The figure shows three views and two pictorial views of one solid part (mm, origin at its lowest corner). Answer the questions. Give positions to 0.01 mm unless a question says otherwise; leave off trailing zeros. Order: outer loops, then holes, each group sorted by start corner. A loop starts at its lowest first (then second) coordinate and runs counter-clockwise, first axis right, second up. Notation, with made-up numbers: (-40, 52.25) - (10, 52.25) arc R10 cw to (10, 66.25) - close; hole circle Ø6 at (43, 76). An arc over 180 degrees is marked (long way). Answer as CSV lines item,"result". Start each with the question number.
1. Consider line 1 along Z through (x, y) = (7.5, 3); line 2 along Z through (x, y) = (10.5, 3.25); line 3 along X through (y, z) = (7, 6). Determine where each line is inside the solid, lowest interval first. Write a range as [from, to].
2. A flat-ended cylindrical pin translates along its axis: pin 1 (4 mm diameter, centred on x = 3.5, z = 11, fed in from -Y). Find the tip coordinate at first contact, or state that the pin passes through.
3. Section D-D on x = 1.5 is taken. Give the vertices of the cut face in (y, z).
4. Section C-C on y = 1.75 is taken. Give the vertices of the cut face in (x, z).
5. Determine the mould class of the marked faces 1, 2 and 3 for opening direction X: +X half, -X half, draft (parallel to the pull), parting line (faces both ways), or undercut.
6. Section A-A on z = 32.5 is taken. Give the vertices of the cut face in (x, y), and give its area (4 significant figures).
7. Section B-B on x = 7.5 is taken. Give the vertices of the cut face in (y, z).
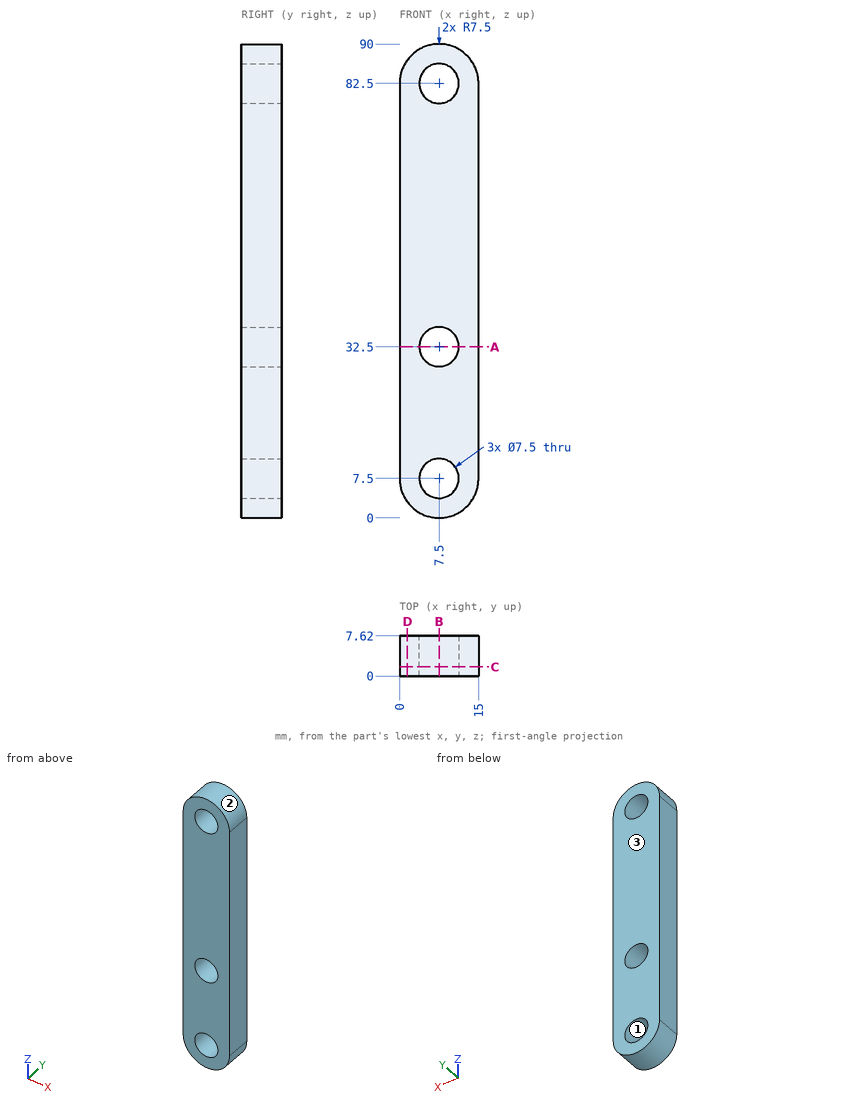
Checks:
1,line 1,"z = [0, 3.75], [11.25, 28.75], [36.25, 78.75], [86.25, 90]"
1,line 2,"z = [0.63, 5.25], [9.75, 30.25], [34.75, 80.25], [84.75, 89.37]"
1,line 3,"x = [0.15, 4.06], [10.94, 14.85]"
2,pin 1,"stops at y = 0"
3,outline,"(0, 3) - (7.62, 3) - (7.62, 87) - (0, 87) - close"
4,outline,"(0, 7.5) arc R7.5 ccw to (15, 7.5) - (15, 82.5) arc R7.5 ccw to (0, 82.5) - close; hole circle Ø7.5 at (7.5, 7.5); hole circle Ø7.5 at (7.5, 32.5); hole circle Ø7.5 at (7.5, 82.5)"
5,face 1,"undercut"
5,face 2,"parting line"
5,face 3,"draft"
6,outline,"(0, 0) - (3.75, 0) - (3.75, 7.62) - (0, 7.62) - close; (11.25, 0) - (15, 0) - (15, 7.62) - (11.25, 7.62) - close"
6,area,"57.15 mm²"
7,outline,"(0, 0) - (7.62, 0) - (7.62, 3.75) - (0, 3.75) - close; (0, 11.25) - (7.62, 11.25) - (7.62, 28.75) - (0, 28.75) - close; (0, 36.25) - (7.62, 36.25) - (7.62, 78.75) - (0, 78.75) - close; (0, 86.25) - (7.62, 86.25) - (7.62, 90) - (0, 90) - close"
